from build123d import *

# Parameters (mm, degrees)
F0_W     = 30
F0_H     = 35
F0_R     = 5.5
F1_DEPTH = 10
F2_R     = 13
F3_SIZE  = 2
F4_SIZE  = 1
F5_SIZE  = 1


with BuildPart() as f1:
    # F0 (on Front) → F1 (new body)
    with BuildSketch(Plane.XZ):
        Rectangle(F0_W, F0_H)
        with Locations((0, -2.5)):
            Circle(F0_R, mode=Mode.SUBTRACT)
    extrude(amount=F1_DEPTH)

    # F2
    f2_edges = [f1.edges().sort_by_distance(p)[0] for p in [
        (15, -5, -17.5),
        (-15, -5, -17.5),
    ]]
    fillet(f2_edges, radius=F2_R)

    # F3
    f3_edges = [f1.edges().sort_by_distance(p)[0] for p in [
        (15, -5, 17.5),
        (-15, -5, 17.5),
        (0, 0, 17.5),
        (0, -10, 17.5),
    ]]
    chamfer(f3_edges, length=F3_SIZE)

    # F4
    f4_edges = [f1.edges().sort_by_distance(p)[0] for p in [
        (-15, -10, 5.5),
        (-15, 0, 5.5),
    ]]
    chamfer(f4_edges, length=F4_SIZE)

    # F5
    f5_edges = [f1.edges().sort_by_distance(p)[0] for p in [
        (5.5, -5, -2.5),
        (-5.5, 0, -2.5),
        (-5.5, -10, -2.5),
    ]]
    chamfer(f5_edges, length=F5_SIZE)


solid = f1.part
Geometry check sheet. Reference: the model listing, model coordinates, mm. Coordinates: 2 decimals unless noted, no trailing zeros. Order: outer loops, then holes, each group sorted by start corner. A loop starts at its lowest first (then second) coordinate and runs counter-clockwise, first axis right, second up. Notation, with made-up numbers: (56.25, 64) - (85.25, 64) arc R27 cw to (85.25, 80) - close; hole circle Ø1 at (-0.5, 61). An arc over 180 degrees is marked (long way). One line per item, written item: value.
(1) Depth check by flat-ended pin: pin 1 Ø1.5 at (x, y) = (6.5, -2) entering from -Z; pin 2 Ø5 at (x, y) = (-3.5, -8.5) entering from -Z. Enter the tip coordinate at first touch or a pass-through.
Data:
pin 1: stops at z = -16.95
pin 2: stops at z = -17.5
(2) Sectioned sample at B-B (x = 0). Enter the section's corners in (y, z), and give its area (3 significant figures).
Data:
outline: (-10, -16.5) - (-9, -17.5) - (-1, -17.5) - (0, -16.5) - (0, -9) - (-1, -8) - (-9, -8) - (-10, -9) - close; (-10, 4) - (-9, 3) - (-1, 3) - (0, 4) - (0, 15.5) - (-2, 17.5) - (-8, 17.5) - (-10, 15.5) - close
area: 233 mm^2
(3) Thickness scan on probe 1 along Z at (x, y) = (0, -3.25); probe 2 along Z at (x, y) = (1, -1); probe 3 along X at (y, z) = (-0.75, -7). Record the ranges inside material, lowest first. Write a range as from..to.
Data:
probe 1: z = -17.5..-8, 3..17.5
probe 2: z = -17.5..-7.91, 2.91..16.5
probe 3: x = -14.5..-3.58, 3.58..14.5
(4) Sectioned sample at A-A (z = -2.5). Enter the section's corners in (x, y).
Data:
outline: (-15, -9) - (-14, -10) - (-6.5, -10) - (-5.5, -9) - (-5.5, -1) - (-6.5, 0) - (-14, 0) - (-15, -1) - close; (5.5, -9) - (6.5, -10) - (14, -10) - (15, -9) - (15, -1) - (14, 0) - (6.5, 0) - (5.5, -1) - close
(5) Release check for a two-part mould opening along X. For faces 1 (the face through (-14.5, -9.5, 5.6)), 2 (the face through (-4.4, -4.9, -5.8)), 3 (the face through (-0.2, -9, 16.5)) record: +X half, -X half, draft (parallel to the pull), parting line (faces both ways), or undercut.
Data:
face 1: -X half
face 2: undercut
face 3: draft
(6) Sectioned sample at C-C (y = -2.75). Enter the section's corners in (x, z), and give its area (3 significant figures).
Data:
outline: (-15, -4.5) arc R13 ccw to (-2, -17.5) - (2, -17.5) arc R13 ccw to (15, -4.5) - (15, 15.5) - (13, 17.5) - (-13, 17.5) - (-15, 15.5) - close; hole circle Ø11 at (0, -2.5)
area: 878 mm^2
